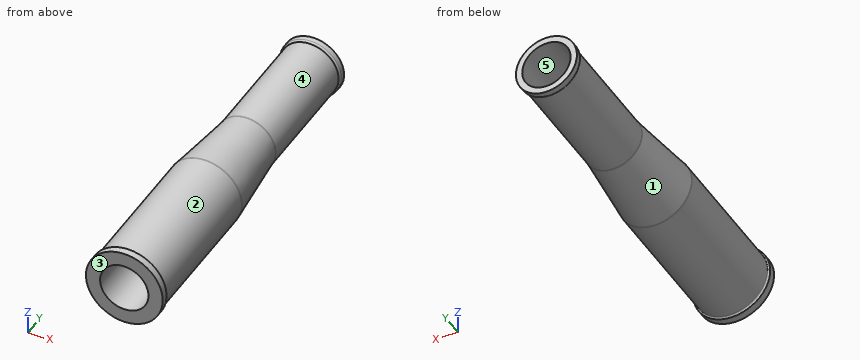
from build123d import *

# Parameters (mm, degrees)
CROQUIS1_R              = 35
SALIENTE_EXTRUIR1_DEPTH = 145
CROQUIS2_R              = 27.5
CROQUIS3_R              = 27.5
SALIENTE_EXTRUIR2_DEPTH = 120
CROQUIS5_R              = 36.5
SALIENTE_EXTRUIR3_DEPTH = 7
CROQUIS4_R              = 23
CORTAR_EXTRUIR1_DEPTH   = 525
REDONDEO1_R             = 10
SALIENTE_EXTRUIR4_START = -7
CROQUIS6_R              = 29
CROQUIS6_R_2            = 23
SALIENTE_EXTRUIR4_DEPTH = 7
REDONDEO2_R             = 2


with BuildPart() as part:
    # Croquis1 → Saliente-Extruir1 (new body)
    with BuildSketch(Plane(origin=(0, 0, 0), x_dir=(1, 0, 0), z_dir=(0, 1, 0))):
        with Locations(Location((0, 0, 0), (0, 0, 270))):
            Circle(CROQUIS1_R)
    extrude(amount=SALIENTE_EXTRUIR1_DEPTH)

    # Croquis2 → section 1 of recubrir1
    with BuildSketch(Plane(origin=(0, 220, 0), x_dir=(1, 0, 0), z_dir=(0, 1, 0)), mode=Mode.PRIVATE) as recubrir1_s1:
        Circle(CROQUIS2_R)
    # loft up to a face of the part (recubrir1)
    loft([Face(Wire([part.edges().sort_by_distance((25.51390196, 145, -23.959148708))[0]])), recubrir1_s1.sketch])

    # Croquis3 → Saliente-Extruir2 (add)
    with BuildSketch(Plane(origin=(0, 220, 0), x_dir=(1, 0, 0), z_dir=(0, 1, 0))):
        with Locations(Location((0, 0, 0), (0, 0, 270))):
            Circle(CROQUIS3_R)
    extrude(amount=SALIENTE_EXTRUIR2_DEPTH)

    # Croquis5 → Saliente-Extruir3 (add)
    with BuildSketch(Plane.XZ):
        with Locations(Location((0, 0, 0), (0, 0, 270))):
            Circle(CROQUIS5_R)
    extrude(amount=-SALIENTE_EXTRUIR3_DEPTH)

    # Croquis4 → Cortar-Extruir1 (cut)
    with BuildSketch(Plane.XZ):
        with Locations(Location((0, 0, 0), (0, 0, 270))):
            Circle(CROQUIS4_R)
    extrude(amount=-CORTAR_EXTRUIR1_DEPTH, mode=Mode.SUBTRACT)

    # Redondeo1
    # the kernel refuses this fillet: 10 mm, written as the material it adds along each edge
    with BuildSketch(Plane(origin=(0, 220, 0), x_dir=(0, 0, 1), z_dir=(1, 0, 0))) as redondeo1_piece_1:
        with BuildLine():
            CenterArc((27.5 + REDONDEO1_R, -REDONDEO1_R * 0.0498756211209), REDONDEO1_R, 174.289406863, 5.710593137)
            Line((27.5 + REDONDEO1_R * 0.00496280979001, REDONDEO1_R * 0.0496280979001), (27.5, 0))
            Line((27.5, 0), (27.5, -REDONDEO1_R * 0.0498756211209))
        make_face()
    revolve(axis=Axis((0, 220, 0), (0, -1, 0)))
    # the kernel refuses this fillet: 10 mm, written as the material it takes off along each edge
    with BuildSketch(Plane(origin=(0, 145, 0), x_dir=(0, 0, 1), z_dir=(-1, 0, 0))) as redondeo1_2_piece_1:
        with BuildLine():
            CenterArc((35 - REDONDEO1_R, -REDONDEO1_R * 0.0498756211209), REDONDEO1_R, 0, 5.710593137)
            Line((35 - REDONDEO1_R * 0.00496280979001, REDONDEO1_R * 0.0496280979001), (35, 0))
            Line((35, 0), (35, -REDONDEO1_R * 0.0498756211209))
        make_face()
    revolve(axis=Axis((0, 145, 0), (0, 1, 0)), mode=Mode.SUBTRACT)

    # Croquis6 → Saliente-Extruir4 (add)
    with BuildSketch(Plane(origin=(0, 340, 0), x_dir=(1, 0, 0), z_dir=(0, 1, 0)).offset(SALIENTE_EXTRUIR4_START)):
        with Locations(Location((0, 0, 0), (0, 0, 270))):
            Circle(CROQUIS6_R)
        with Locations(Location((0, 0, 0), (0, 0, 90))):
            Circle(CROQUIS6_R_2, mode=Mode.SUBTRACT)
    extrude(amount=SALIENTE_EXTRUIR4_DEPTH)

    # Redondeo2
    # the kernel refuses this fillet: 2 mm, written as the material it adds along each edge
    with BuildSketch(Plane(origin=(0, 7, 0), x_dir=(0, 0, 1), z_dir=(1, 0, 0))) as redondeo2_piece_1:
        with BuildLine():
            CenterArc((37, -1.936491673), REDONDEO2_R, 104.477512186, 75.522487814)
            Line((35, -1.936491673), (34.96, -1.936491673))
            Line((34.96, -1.936491673), (34.96, 0))
            Line((34.96, 0), (35, 0.04))
            ThreePointArc((35, 0.04), (35.75, 0.04), (36.49, 0.038729833))
            Line((36.49, 0.038729833), (36.5, 0))
        make_face()
    revolve(axis=Axis((0, 7, 0), (0, -1, 0)))
    # the kernel refuses this fillet: 2 mm, written as the material it takes off along each edge
    with BuildSketch(Plane(origin=(0, 333, 0), x_dir=(0, 0, 1), z_dir=(-1, 0, 0))) as redondeo2_2_piece_1:
        with BuildLine():
            CenterArc((27, 1.936491673), REDONDEO2_R, 284.477512186, 75.522487814)
            Line((29, 1.936491673), (29.04, 1.936491673))
            Line((29.04, 1.936491673), (29.04, 0))
            Line((29.04, 0), (29, -0.04))
            ThreePointArc((29, -0.04), (28.25, -0.04), (27.51, -0.038729833))
            Line((27.51, -0.038729833), (27.5, 0))
        make_face()
    revolve(axis=Axis((0, 333, 0), (0, 1, 0)), mode=Mode.SUBTRACT)


solid = part.part
Verification items for the finished model (mm, model axes). Face numbers are marked on the shaded views. A direction names the side the tool comes from. Give positions to 0.01 mm unless a question says otherwise; leave off trailing zeros. Loops run counter-clockwise (first coordinate to the right, second up) from the corner with the lowest first, then second, coordinate; pieces in that order, holes last.
1) Depth check by flat-ended pin: pin 1 Ø10 at (x, y) = (-5, 146) entering from -Z; pin 2 Ø5 at (x, y) = (7.5, 167) entering from -Z; pin 3 Ø2 at (x, y) = (10.5, 72.5) entering from +Z. Enter the tip coordinate at first touch or a pass-through.
2) Sectioned sample at C-C, the plane y = 202. Enter the section's corners in (x, z), then the cut area to 3 significant figures.
3) Draft check along X on the marked faces 3, 4 and 5. Enter one of: pulls with the +X half, pulls with the -X half, needs draft (parallel to the pull), parting line crosses it, or undercut.
4) Set-up check for the marked faces 1 and 2: record each of +Z, -Z, +X, -X, +Y, -Y from which the full face is reachable in a straight line by a thin tool's end or side.
5) Sectioned sample at A-A, the plane z = 0. Enter the section's corners in (x, y).
6) Thickness scan on line 1 along X through (y, z) = (155, 18); line 2 along X through (y, z) = (94.5, -16); line 3 along Z through (x, y) = (3.5, 29). Record the ranges inside material, lowest first.
7) Sectioned sample at B-B, the plane y = 139. Enter the section's corners in (x, z), then the cut area to 3 significant figures.
Answers:
1. pin 1: stops at z = -35
1. pin 2: stops at z = -32.49
1. pin 3: stops at z = 33.69
2. outline: circle Ø58.6 at (0, 0); hole circle Ø46 at (0, 0)
2. area: 1,040 mm2
3. face 3: needs draft
3. face 4: parting line crosses it
3. face 5: undercut
4. face 1: none
4. face 2: +Y
5. outline: (-36.5, 0) - (-23, 0) - (-23, 340) - (-29, 340) - (-29, 334.94) arc R2 ccw to (-27.5, 333) - (-27.5, 220.5) arc R10 cw to (-27.55, 219.5) - (-34.95, 145.5) arc R10 ccw to (-35, 144.5) - (-35, 8.94) arc R2 cw to (-36.5, 7) - close; (23, 0) - (36.5, 0) - (36.5, 7) arc R2 cw to (35, 8.94) - (35, 144.5) arc R10 ccw to (34.95, 145.5) - (27.55, 219.5) arc R10 cw to (27.5, 220.5) - (27.5, 333) arc R2 ccw to (29, 334.94) - (29, 340) - (23, 340) - close
6. line 1: x = -28.84 to -14.32, 14.32 to 28.84
6. line 2: x = -31.13 to -16.52, 16.52 to 31.13
6. line 3: z = -34.82 to -22.73, 22.73 to 34.82
7. outline: circle Ø70 at (0, 0); hole circle Ø46 at (0, 0)
7. area: 2,190 mm2
